Model file for the job. Use its own axes, mm. A direction names the side the tool comes from. Give positions to 0.01 mm unless a question says otherwise; leave off trailing zeros. Write each loop counter-clockwise with the first axis right and the second up, starting at its lowest first coordinate (ties: lowest second). Pieces come first, ordered by that corner, then holes. Notation, with made-up numbers: (-39, 55) - (3, 55) arc R25 ccw to (3, 77) - close; hole circle Ø10 at (18.25, 57). An arc over 180 degrees is marked (long way). One line per item, written item: value. Start each with the question number.
(1) 3-axis set-ups, long thin cutter, end or side, ignore diameter. For faces 1 (the face through (40, 15, 304.8)), 2 (the face through (38.1, 22, 150)): which of +Z, -Z, +X, -X, +Y, -Y reach the whole face in a straight line?
(2) Probe L1, parallel to Y at x = 32.5, z = 43 (3 decimals); L2, parallel to X at y = 4, z = 263 (3 decimals); L3, parallel to Z at x = 38.5, y = 13.5. List the from-to ranges inside material, lowest first.
(3) Drop flat-ended pins along their axis: P1, Ø8, axis at x = 13.5, z = 261.5, coming from the +Y side (3 decimals); P2, Ø3, axis at y = 19, z = 80.5, coming from the -X side. Give the stop position or say it passes through.
(4) Cut at C-C, the plane z = 193. List the corners of the cut face in (x, y) (3 decimals), and give its area (3 significant figures).
(5) Cut at B-B, the plane y = 35.5. List the corners of the cut face in (x, z) (3 decimals).
(6) Cut at A-A, the plane x = 31.5. List the corners of the cut face in (y, z) (3 decimals).
(7) Cut at D-D, the plane x = 18.5. List the corners of the cut face in (y, z) (3 decimals).
from build123d import *

# Parameters (mm, degrees)
F1_DEPTH     = 304.8
F2_R         = 0.762
F5_DEPTH     = 25.4
F6_R         = 0.381
F7_T1_DEPTH  = 3.175
F7_T4_ANGLE  = 90
F7_T6_ANGLE  = 90
F7_T8_ANGLE  = 90
F7_T10_ANGLE = 90


# Not quite as in the source:
# - a fillet or chamfer that OpenCascade refuses, or shapes differently, is made with other operations: its cross-section is extruded or revolved along the edge and cut away or added


with BuildPart() as f1:
    # F0 (on Top) → F1 (new body)
    with BuildSketch(Plane.XY):
        Polygon((0, 3.175), (0, 0), (41.275, 0), (41.275, 41.275), (38.1, 41.275), (38.1, 3.175), align=None)
    extrude(amount=F1_DEPTH)

    # F2
    f2_edges = [f1.edges().sort_by_distance(p)[0] for p in [
        (0, 0, 152.4),
        (20.6375, 0, 304.8),
        (20.6375, 0, 0),
        (38.1, 22.225, 304.8),
        (19.05, 3.175, 304.8),
        (0, 3.175, 152.4),
        (19.05, 3.175, 0),
        (38.1, 22.225, 0),
        (38.1, 41.275, 152.4),
    ]]
    fillet(f2_edges, radius=F2_R)

    # F4 (on face) → F5 (cut)
    with BuildSketch(Plane.XZ):
        with BuildLine():
            ThreePointArc((27.178, 159.5842048969), (20.6375, 162.1155), (14.097, 159.5842048969))
            Line((14.097, 159.5842048969), (14.097, 145.2157951031))
            ThreePointArc((14.097, 145.2157951031), (20.6375, 142.6845), (27.178, 145.2157951031))
            Line((27.178, 145.2157951031), (27.178, 159.5842048969))
        make_face()
    extrude(amount=-F5_DEPTH, mode=Mode.SUBTRACT)

    # F6
    f6_edges = [f1.edges().sort_by_distance(p)[0] for p in [
        (14.097, 1.5875, 145.215795),
        (14.097, 1.5875, 159.584205),
        (27.178, 1.5875, 159.584205),
        (27.178, 1.5875, 145.215795),
    ]]
    fillet(f6_edges, radius=F6_R)

    # F7: fillet of radius 12.7 on 2 edges, made by hand

    # F7_s2 → F7_t1 (cut)
    with BuildSketch(Plane.XZ.offset(-3.175)):
        with BuildLine():
            ThreePointArc((12.7, 304.8), (3.7197438789, 301.0802561211), (0, 292.1))
            Line((0, 292.1), (0, 304.8))
            Line((0, 304.8), (12.7, 304.8))
        make_face()
        with BuildLine():
            ThreePointArc((12.7, 0), (3.7197438789, 3.7197438789), (0, 12.7))
            Line((0, 12.7), (0, 0))
            Line((0, 0), (12.7, 0))
        make_face()
    extrude(amount=F7_T1_DEPTH, mode=Mode.SUBTRACT)

    # F7_s3 → F7_t4 (revolve, cut)
    with BuildSketch(Plane.YZ.offset(12.7)):
        with BuildLine():
            ThreePointArc((3.175, 0.762), (2.9518153673, 0.2231846327), (2.413, 0))
            Line((2.413, 0), (3.175, 0))
            Line((3.175, 0), (3.175, 0.762))
        make_face()
    revolve(axis=Axis((12.7, 3.175, 12.7), (0, 1, 0)), revolution_arc=F7_T4_ANGLE, mode=Mode.SUBTRACT)

    # F7_s5 → F7_t6 (revolve, cut)
    with BuildSketch(Plane.XY.offset(12.7)):
        with BuildLine():
            ThreePointArc((0.762, 0), (0.2231846327, 0.2231846327), (0, 0.762))
            Line((0, 0.762), (0, 0))
            Line((0, 0), (0.762, 0))
        make_face()
    revolve(axis=Axis((12.7, 0, 12.7), (0, -1, 0)), revolution_arc=F7_T6_ANGLE, mode=Mode.SUBTRACT)

    # F7_s7 → F7_t8 (revolve, cut)
    with BuildSketch(Plane.XY.offset(292.1)):
        with BuildLine():
            ThreePointArc((0.762, 3.175), (0.2231846327, 2.9518153673), (0, 2.413))
            Line((0, 2.413), (0, 3.175))
            Line((0, 3.175), (0.762, 3.175))
        make_face()
    revolve(axis=Axis((12.7, 3.175, 292.1), (0, 1, 0)), revolution_arc=F7_T8_ANGLE, mode=Mode.SUBTRACT)

    # F7_s9 → F7_t10 (revolve, cut)
    with BuildSketch(Plane.YZ.offset(12.7)):
        with BuildLine():
            ThreePointArc((0, 304.038), (0.2231846327, 304.5768153673), (0.762, 304.8))
            Line((0.762, 304.8), (0, 304.8))
            Line((0, 304.8), (0, 304.038))
        make_face()
    revolve(axis=Axis((12.7, 0, 292.1), (0, -1, 0)), revolution_arc=F7_T10_ANGLE, mode=Mode.SUBTRACT)


solid = f1.part
Answers follow:
1. face 1: +Z, +X, -X, +Y, -Y
1. face 2: +Z, -Z, -X, +Y
2. L1: y = 0 to 3.175
2. L2: x = 38.1 to 41.275
2. L3: z = 0.09 to 304.71
3. P1: stops at y = 3.175
3. P2: stops at x = 38.1
4. outline: (0, 0.762) arc R0.762 ccw to (0.762, 0) - (41.275, 0) - (41.275, 41.275) - (38.862, 41.275) arc R0.762 ccw to (38.1, 40.513) - (38.1, 3.175) - (0.762, 3.175) arc R0.762 ccw to (0, 2.413) - close
4. area: 252 mm²
5. outline: (38.1, 0.762) arc R0.762 ccw to (38.862, 0) - (41.275, 0) - (41.275, 304.8) - (38.862, 304.8) arc R0.762 ccw to (38.1, 304.038) - close
6. outline: (0, 0.762) arc R0.762 ccw to (0.762, 0) - (2.413, 0) arc R0.762 ccw to (3.175, 0.762) - (3.175, 304.038) arc R0.762 ccw to (2.413, 304.8) - (0.762, 304.8) arc R0.762 ccw to (0, 304.038) - close
7. outline: (0, 0.762) arc R0.762 ccw to (0.762, 0) - (2.413, 0) arc R0.762 ccw to (3.175, 0.762) - (3.175, 142.923) - (0, 142.923) - close; (0, 161.877) - (3.175, 161.877) - (3.175, 304.038) arc R0.762 ccw to (2.413, 304.8) - (0.762, 304.8) arc R0.762 ccw to (0, 304.038) - close
